Read the model definition and answer for the solid it produces. Units are mm, in the model's axes. Face numbers are marked on the shaded views. A direction names the side the tool comes from. Round coordinates to 2 decimals unless told otherwise and drop trailing zeros. Order: outer loops, then holes, each group sorted by start corner. A loop starts at its lowest first (then second) coordinate and runs counter-clockwise, first axis right, second up. Notation, with made-up numbers: (-1, 2) - (16, 2) arc R16 ccw to (16, 28) - close; hole circle Ø7 at (10.25, 30). An arc over 180 degrees is marked (long way). Put each result on its own line as item: value. Start each with the question number.
Q1. Which of the six approach directions +Z, -Z, +X, -X, +Y, -Y give full straight-line access (tool end or side, diameter ignored) to the marked faces 1, 2 and 3?
Q2. Section D-D on x = 22.5 is taken. Give the vertices of the cut face in (y, z), then the cut area to 3 significant figures.
Q3. Section B-B on x = 7 is taken. Give the vertices of the cut face in (y, z).
Q4. Find the intervals of material crossed by line 1 along X through (y, z) = (0.65, -7); line 2 along Z through (x, y) = (22.5, 23.55); line 3 along Z through (x, y) = (18, 37), in increasing order. Write a range as from..to.
Q5. Section C-C on z = -22.5 is taken. Give the vertices of the cut face in (x, y), then the cut area to 3 significant figures.
Q6. Each of these flat-tipped pins is pushed along its axis until it touches: pin 1 Ø1.5 at (x, y) = (17, 26.5) entering from -Z; pin 2 Ø1.5 at (x, y) = (23.5, 21) entering from +Z; pin 3 Ø2.5 at (x, z) = (22.5, 5) entering from -Y; pin 4 Ø3.5 at (x, z) = (22.5, 5) entering from +Y. Where does it stop, or does it pass through?
Q7. Section A-A on z = -7 is taken. Give the vertices of the cut face in (x, y), then the cut area to 3 significant figures.
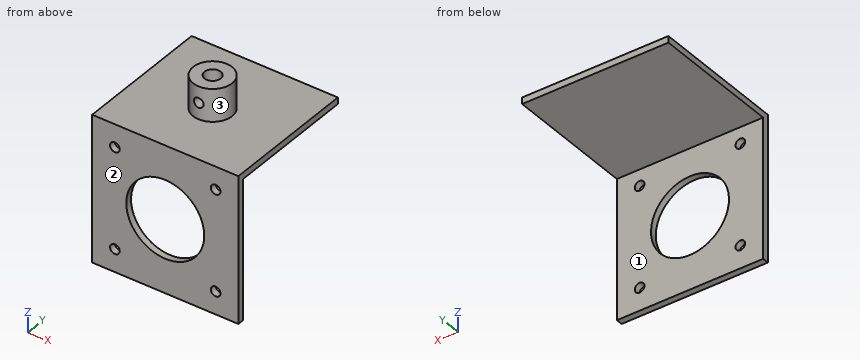
from build123d import *

# Parameters (mm, degrees)
SKETCH_1_W               = 45
SKETCH_1_H               = 45
EXTRUDE_1_DEPTH          = 2
SKETCH_3_R               = 12
SKETCH_3_R_2             = 1.5
CUT_EXTRUDE_1_DEPTH      = 10
SKETCH_7_W               = 45
SKETCH_7_H               = 2
EXTRUDE_3_DEPTH          = 40
SKETCH_8_R               = 6
SKETCH_8_R_2             = 2.5
EXTRUDE_4_DEPTH          = 10
CUT_EXTRUDE_2_DEPTH      = 77.249590163
CUT_EXTRUDE_2_DEPTH_BACK = 77.249590163
SKETCH_9_R               = 1.5


with BuildPart() as part:
    # 草图1 → 凸台-拉伸1 (new body)
    with BuildSketch(Plane(origin=(0, 0, 0), x_dir=(1, 0, 0), z_dir=(0, 1, 0))):
        with Locations((22.5, 22.5)):
            Rectangle(SKETCH_1_W, SKETCH_1_H)
    extrude(amount=EXTRUDE_1_DEPTH)

    # 草图3 → 切除-拉伸1 (cut)
    with BuildSketch(Plane(origin=(0, 2, 0), x_dir=(1, 0, 0), z_dir=(0, 1, 0))):
        with Locations(Location((22.5, 22.5, 0), (0, 0, 270))):
            Circle(SKETCH_3_R)
        with Locations(Location((38, 38, 0), (0, 0, 270))):
            Circle(SKETCH_3_R_2)
        with Locations(Location((7, 38, 0), (0, 0, 270))):
            Circle(SKETCH_3_R_2)
        with Locations(Location((7, 7, 0), (0, 0, 270))):
            Circle(SKETCH_3_R_2)
        with Locations(Location((38, 7, 0), (0, 0, 270))):
            Circle(SKETCH_3_R_2)
    extrude(amount=-CUT_EXTRUDE_1_DEPTH, mode=Mode.SUBTRACT)

    # 草图7 → 凸台-拉伸3 (add)
    with BuildSketch(Plane(origin=(0, 2, 0), x_dir=(1, 0, 0), z_dir=(0, 1, 0))):
        with Locations((22.5, 1)):
            Rectangle(SKETCH_7_W, SKETCH_7_H)
    extrude(amount=EXTRUDE_3_DEPTH)

    # 草图8 → 凸台-拉伸4 (add)
    with BuildSketch(Plane.XY):
        with Locations((22.5, 20)):
            Circle(SKETCH_8_R)
        with Locations((22.5, 20)):
            Circle(SKETCH_8_R_2, mode=Mode.SUBTRACT)
    extrude(amount=EXTRUDE_4_DEPTH)

    # 草图9 → 切除-拉伸2 (cut, two sides: drawn at the far end of the back side and taken through both)
    with BuildSketch(Plane(origin=(0, 0, 0), x_dir=(1, 0, 0), z_dir=(0, 1, 0)).offset(-CUT_EXTRUDE_2_DEPTH_BACK)):
        with Locations(Location((22.5, -5, 0), (0, 0, 270))):
            Circle(SKETCH_9_R)
    extrude(amount=CUT_EXTRUDE_2_DEPTH + CUT_EXTRUDE_2_DEPTH_BACK, mode=Mode.SUBTRACT)


solid = part.part
Findings:
1. face 1: -Z, +X, -X, +Y
1. face 2: +Z, -Z, +X, -X, -Y
1. face 3: +Z
2. outline: (0, -45) - (2, -45) - (2, -34.5) - (0, -34.5) - close; (0, -10.5) - (2, -10.5) - (2, -2) - (42, -2) - (42, 0) - (26, 0) - (26, 3.5) - (22.5, 3.5) - (22.5, 0) - (17.5, 0) - (17.5, 3.5) - (14, 3.5) - (14, 0) - (0, 0) - close; (14, 6.5) - (17.5, 6.5) - (17.5, 10) - (14, 10) - close; (22.5, 6.5) - (26, 6.5) - (26, 10) - (22.5, 10) - close
2. area: 171 mm2
3. outline: (0, -45) - (2, -45) - (2, -39.5) - (0, -39.5) - close; (0, -36.5) - (2, -36.5) - (2, -8.5) - (0, -8.5) - close; (0, -5.5) - (2, -5.5) - (2, -2) - (42, -2) - (42, 0) - (0, 0) - close
4. line 1: 0..5.5, 8.5..36.5, 39.5..45
4. line 2: -2..3.5, 6.5..10
4. line 3: -2..0
5. outline: (0, 0) - (10.5, 0) - (10.5, 2) - (0, 2) - close; (34.5, 0) - (45, 0) - (45, 2) - (34.5, 2) - close
5. area: 42.0 mm2
6. pin 1: z = -2
6. pin 2: z = 0
6. pin 3: through
6. pin 4: y = 26
7. outline: (0, 0) - (5.5, 0) - (5.5, 2) - (0, 2) - close; (8.5, 0) - (36.5, 0) - (36.5, 2) - (8.5, 2) - close; (39.5, 0) - (45, 0) - (45, 2) - (39.5, 2) - close
7. area: 78.0 mm2
